Design review of the part built by this model. Coordinates are the model's own, in mm. A direction names the side the tool comes from. Coordinates: 2 decimals unless noted, no trailing zeros. Write each loop counter-clockwise with the first axis right and the second up, starting at its lowest first coordinate (ties: lowest second). Pieces come first, ordered by that corner, then holes. Notation, with made-up numbers: (-39.75, 8.5) - (14.25, 8.5) arc R19 ccw to (14.25, 41.5) - close; hole circle Ø4 at (20.25, 87.25). An arc over 180 degrees is marked (long way). One line per item, written item: value.
from build123d import *

# Parameters (mm, degrees)
SKETCH1_W           = 18
SKETCH1_H           = 18
SKETCH1_W_2         = 16.4
SKETCH1_H_2         = 16.4
BOSS_EXTRUDE1_DEPTH = 34
SKETCH2_W           = 18
SKETCH2_H           = 18
BOSS_EXTRUDE2_DEPTH = 1.2
CHAMFER1_SIZE       = 0.5


with BuildPart() as part:
    # Sketch1 → Boss-Extrude1 (new body)
    with BuildSketch(Plane(origin=(0, 0, 0), x_dir=(1, 0, 0), z_dir=(0, 1, 0))):
        Rectangle(SKETCH1_W, SKETCH1_H)
        Rectangle(SKETCH1_W_2, SKETCH1_H_2, mode=Mode.SUBTRACT)
    extrude(amount=BOSS_EXTRUDE1_DEPTH)

    # Sketch2 → Boss-Extrude2 (add)
    with BuildSketch(Plane(origin=(0, 34, 0), x_dir=(1, 0, 0), z_dir=(0, 1, 0))):
        Rectangle(SKETCH2_W, SKETCH2_H)
    extrude(amount=BOSS_EXTRUDE2_DEPTH)

    # Chamfer1
    chamfer1_edges = [part.edges().sort_by_distance(p)[0] for p in [
        (-9, 35.2, 0),
        (0, 35.2, 9),
        (9, 35.2, 0),
        (0, 35.2, -9),
    ]]
    chamfer(chamfer1_edges, length=CHAMFER1_SIZE)


solid = part.part
1. Consider section B-B, the plane x = -3.25. Write out the cut boundary in (y, z).
Answer block:
outline: (0, -9) - (34.7, -9) - (35.2, -8.5) - (35.2, 8.5) - (34.7, 9) - (0, 9) - (0, 8.2) - (34, 8.2) - (34, -8.2) - (0, -8.2) - close
2. For faces 4 (the face through (0, 34, 0)), 5 (the face through (9, 17, 0)), list the 3-axis set-ups (+Z, -Z, +X, -X, +Y, -Y) from which the entire face can be reached by the end or side of a thin tool; tool diameter is ignored.
Answer block:
face 4: -Y
face 5: +Z, -Z, +X, +Y, -Y
3. Mouldability with a two-part tool opening along Z and no side actions: class faces 1 (the face through (-8.2, 17, 0)), 2 (the face through (0, 35.2, 0)), 3 (the face through (0, 17, -9)) as released by +Z, released by -Z, zero draft, split by the parting line, or undercut.
Answer block:
face 1: undercut
face 2: zero draft
face 3: released by -Z
4. Consider section A-A, the plane y = 26. Write out the cut boundary in (x, z).
Answer block:
outline: (-9, -9) - (9, -9) - (9, 9) - (-9, 9) - close; hole (-8.2, -8.2) - (8.2, -8.2) - (8.2, 8.2) - (-8.2, 8.2) - close
5. Insertion check: pin 1 Ø2 at (x, z) = (-0.5, -3) entering from -Y. The pin has a flat end and moves straight along its axis. Give the tip position at first contact, or say it passes through.
Answer block:
pin 1: stops at y = 34
6. Wall thickness on line 1 along X through (y, z) = (22.5, -4); line 2 along Y through (x, z) = (-5.75, -3): over which ranges is each line inside the solid? List them lowest first.
Answer block:
line 1: x = -9 to -8.2, 8.2 to 9
line 2: y = 34 to 35.2
7. Consider section C-C, the plane z = 3. Write out the cut boundary in (x, y).
Answer block:
outline: (-9, 0) - (-8.2, 0) - (-8.2, 34) - (8.2, 34) - (8.2, 0) - (9, 0) - (9, 34.7) - (8.5, 35.2) - (-8.5, 35.2) - (-9, 34.7) - close
